from build123d import *

# Parameters (mm, degrees)
F1_DEPTH = 25.4
F2_R     = 6.35
F3_DEPTH = 25.4
F4_R     = 6.35
F5_DEPTH = 38.1
F7_DEPTH = 25.4


with BuildPart() as f1:
    # F0 (on Front) → F1 (new body)
    with BuildSketch(Plane.XZ):
        Polygon((0, 12.7), (0, 0), (101.6, 0), (101.6, 12.7), (50.8, 12.7), (50.8, 50.8), (25.4, 50.8), (25.4, 12.7), align=None)
    extrude(amount=F1_DEPTH)

    # F2 (on face) → F3 (cut)
    with BuildSketch(Plane.XY.offset(12.7)):
        with Locations((12.7, -12.7)):
            Circle(F2_R)
        with BuildLine():
            ThreePointArc((0, -12.7), (3.719744, -3.719744), (12.7, 0))
            Line((12.7, 0), (0, 0))
            Line((0, 0), (0, -12.7))
        make_face()
        with BuildLine():
            ThreePointArc((12.7, -25.4), (3.719744, -21.680256), (0, -12.7))
            Line((0, -12.7), (0, -25.4))
            Line((0, -25.4), (12.7, -25.4))
        make_face()
    extrude(amount=-F3_DEPTH, mode=Mode.SUBTRACT)

    # F4 (on face) → F5 (cut)
    with BuildSketch(Plane.XY.offset(50.8)):
        with BuildLine():
            ThreePointArc((38.1, 0), (47.080256, -3.719744), (50.8, -12.7))
            Line((50.8, -12.7), (50.8, 0))
            Line((50.8, 0), (38.1, 0))
        make_face()
        with Locations((38.1, -12.7)):
            Circle(F4_R)
        with BuildLine():
            ThreePointArc((25.4, -12.7), (29.119744, -3.719744), (38.1, 0))
            Line((38.1, 0), (25.4, 0))
            Line((25.4, 0), (25.4, -12.7))
        make_face()
        with BuildLine():
            Line((25.4, -25.4), (38.1, -25.4))
            ThreePointArc((38.1, -25.4), (29.119744, -21.680256), (25.4, -12.7))
            Line((25.4, -12.7), (25.4, -25.4))
        make_face()
        with BuildLine():
            Line((50.8, -25.4), (50.8, -12.7))
            ThreePointArc((50.8, -12.7), (47.080256, -21.680256), (38.1, -25.4))
            Line((38.1, -25.4), (50.8, -25.4))
        make_face()
    extrude(amount=-F5_DEPTH, mode=Mode.SUBTRACT)

    # F6 (on face) → F7 (cut)
    with BuildSketch(Plane.XY.offset(12.7)):
        with BuildLine():
            ThreePointArc((88.9, -19.05), (82.55, -12.7), (88.9, -6.35))
            Line((88.9, -6.35), (63.5, -6.35))
            ThreePointArc((63.5, -6.35), (67.990128, -8.209872), (69.85, -12.7))
            ThreePointArc((69.85, -12.7), (67.990128, -17.190128), (63.5, -19.05))
            Line((63.5, -19.05), (88.9, -19.05))
        make_face()
        with BuildLine():
            ThreePointArc((69.85, -12.7), (67.990128, -8.209872), (63.5, -6.35))
            ThreePointArc((63.5, -6.35), (57.15, -12.7), (63.5, -19.05))
            ThreePointArc((63.5, -19.05), (67.990128, -17.190128), (69.85, -12.7))
        make_face()
        with BuildLine():
            ThreePointArc((88.9, -19.05), (93.390128, -17.190128), (95.25, -12.7))
            ThreePointArc((95.25, -12.7), (93.390128, -8.209872), (88.9, -6.35))
            ThreePointArc((88.9, -6.35), (82.55, -12.7), (88.9, -19.05))
        make_face()
        with BuildLine():
            ThreePointArc((101.6, -12.7), (97.880256, -21.680256), (88.9, -25.4))
            Line((88.9, -25.4), (101.6, -25.4))
            Line((101.6, -25.4), (101.6, -12.7))
        make_face()
        with BuildLine():
            ThreePointArc((88.9, 0), (97.880256, -3.719744), (101.6, -12.7))
            Line((101.6, -12.7), (101.6, 0))
            Line((101.6, 0), (88.9, 0))
        make_face()
    extrude(amount=-F7_DEPTH, mode=Mode.SUBTRACT)


solid = f1.part
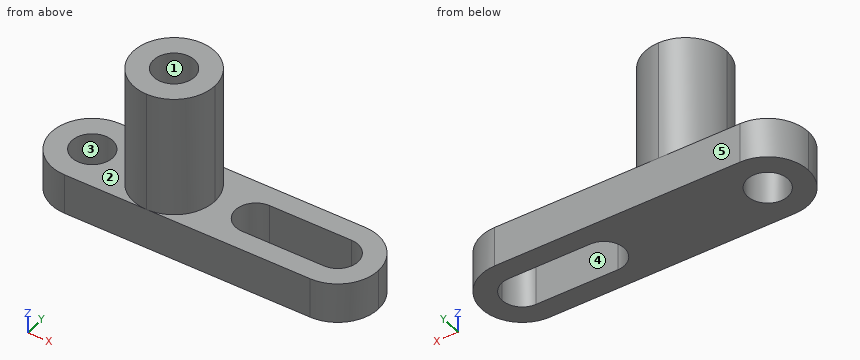
Can you work these out from the model? Positions are in its coordinate system, mm. Face numbers are marked on the shaded views. A direction names the side the tool comes from. Give positions to 0.01 mm unless a question says otherwise; leave off trailing zeros. Loops run counter-clockwise (first coordinate to the right, second up) from the corner with the lowest first, then second, coordinate; pieces in that order, holes last. Notation, with made-up numbers: (-32.75, 50) - (11.25, 50) arc R30 cw to (11.25, 82) - close; hole circle Ø8 at (74.25, -28). An arc over 180 degrees is marked (long way). Return JSON: item names as keys, results as strings.
1. We'd pull the mould along X, two halves only. Please class the marked faces 1, 2 and 3: +X half, -X half, draft (parallel to the pull), parting line (faces both ways), or undercut.
Output values:
{"face 1": "undercut", "face 2": "draft", "face 3": "undercut"}
2. I want a section at A-A on x = 66. Please give me the cut outline in (y, z).
Output values:
{"outline": "(-25.4, 0) - (-19.05, 0) - (-19.05, 12.7) - (-25.4, 12.7) - close; (-6.35, 0) - (0, 0) - (0, 12.7) - (-6.35, 12.7) - close"}
3. I want a section at D-D on z = 33. Please give me the cut outline in (x, y), and give its area (3 significant figures).
Output values:
{"outline": "circle Ø25.4 at (38.1, -12.7); hole circle Ø12.7 at (38.1, -12.7)", "area": "380 mm²"}
4. If I drill on line 1 (X direction, y = -8.25, z = 5); line 2 (Y direction, x = 79, z = 10), over which ranges is the centre line in solid material (lowest first)?
Output values:
{"line 1": "x = 0.81 to 8.17, 17.23 to 58.97, 93.43 to 100.79", "line 2": "y = -25.4 to -19.05, -6.35 to 0"}
5. For the marked faces 4 and 5, which set-ups out of +Z, -Z, +X, -X, +Y, -Y let a thin tool reach every point of the face, with its end or its side?
Output values:
{"face 4": "+Z, -Z", "face 5": "+Z, -Z, +X, -X, +Y"}
6. I want a section at C-C on y = -9.75. Please give me the cut outline in (x, z), and give its area (3 significant figures).
Output values:
{"outline": "(0.35, 0) - (7.08, 0) - (7.08, 12.7) - (0.35, 12.7) - close; (18.32, 0) - (57.88, 0) - (57.88, 12.7) - (50.45, 12.7) - (50.45, 50.8) - (43.72, 50.8) - (43.72, 12.7) - (32.48, 12.7) - (32.48, 50.8) - (25.75, 50.8) - (25.75, 12.7) - (18.32, 12.7) - close; (94.52, 0) - (101.25, 0) - (101.25, 12.7) - (94.52, 12.7) - close", "area": "1,190 mm²"}
7. I'm going to push flat-ended pins straight in: pin 1 Ø6 at (y, z) = (-19, 25.5) entering from +X; pin 2 Ø3 at (x, y) = (56.5, -3.5) entering from +Z; pin 3 Ø1.5 at (y, z) = (-22.5, 10) entering from +X. Where does each tip first touch, or does it pass through?
Output values:
{"pin 1": "stops at x = 50.36", "pin 2": "stops at z = 12.7", "pin 3": "stops at x = 97.81"}
8. I want a section at B-B on z = 5. Please give me the cut outline in (x, y), and give its area (3 significant figures).
Output values:
{"outline": "(12.7, -25.4) - (88.9, -25.4) arc R12.7 ccw to (88.9, 0) - (12.7, 0) arc R12.7 ccw to start; hole circle Ø12.7 at (12.7, -12.7); hole (63.5, -19.05) - (88.9, -19.05) arc R6.35 ccw to (88.9, -6.35) - (63.5, -6.35) arc R6.35 ccw to start", "area": "1,870 mm²"}
